CAD build for the part. Positions are in the model's coordinates, mm. Face numbers are marked on the shaded views. A direction names the side the tool comes from. Give positions to 0.01 mm unless a question says otherwise; leave off trailing zeros. Write each loop counter-clockwise with the first axis right and the second up, starting at its lowest first coordinate (ties: lowest second). Pieces come first, ordered by that corner, then holes. Notation, with made-up numbers: (-20, 65.5) - (17, 65.5) arc R23 ccw to (17, 97.5) - close; hole circle Ø3 at (-12, 27). An arc over 180 degrees is marked (long way). Answer as a JSON object with one key per item and string values.
from build123d import *

# Parameters (mm, degrees)
F0_W      = 24
F0_H      = 24
F1_DEPTH  = 6.5
F4_R      = 4
F5_R      = 1.35
F6_DEPTH  = 6.501
F8_DEPTH  = 5.5
F9_DEPTH  = 6.501
F10_DEPTH = 3.5


with BuildPart() as f1:
    # F0 (on Top) → F1 (new body)
    with BuildSketch(Plane.XY):
        with Locations((12, 12)):
            Rectangle(F0_W, F0_H)
    extrude(amount=F1_DEPTH)

    # F4
    f4_edges = [f1.edges().sort_by_distance(p)[0] for p in [
        (0, 0, 3.25),
        (24, 0, 3.25),
        (24, 24, 3.25),
        (0, 24, 3.25),
    ]]
    fillet(f4_edges, radius=F4_R)

    # F5 (on face) → F6 (cut, through all)
    with BuildSketch(Plane.XY.offset(6.5)):
        with Locations((4, 4)):
            Circle(F5_R)
        with Locations((4, 20)):
            Circle(F5_R)
        with Locations((20, 4)):
            Circle(F5_R)
        with Locations((20, 20)):
            Circle(F5_R)
    extrude(amount=-F6_DEPTH, mode=Mode.SUBTRACT)

    # F7 (on face) → F8 (cut, through all)
    with BuildSketch(Plane.XY.offset(6.5)):
        Polygon((16.1, 3.9), (16.1, 12), (16.1, 20.1), (7.9, 20.1), (7.9, 12), (7.9, 3.9), align=None)
        with BuildLine():
            Line((10.1, 9), (10.1, 15))
            ThreePointArc((10.1, 15), (12, 16.9), (13.9, 15))
            Line((13.9, 15), (13.9, 9))
            ThreePointArc((13.9, 9), (12, 7.1), (10.1, 9))
        make_face(mode=Mode.SUBTRACT)
    extrude(amount=-F8_DEPTH, mode=Mode.SUBTRACT)

    # F7 (on face) → F9 (cut, through all)
    with BuildSketch(Plane.XY.offset(6.5)):
        with BuildLine():
            ThreePointArc((13.9, 15), (12, 16.9), (10.1, 15))
            Line((10.1, 15), (10.1, 9))
            ThreePointArc((10.1, 9), (12, 7.1), (13.9, 9))
            Line((13.9, 9), (13.9, 15))
        make_face()
    extrude(amount=-F9_DEPTH, mode=Mode.SUBTRACT)

    # F7 (on face) → F10 (cut, through all)
    with BuildSketch(Plane.XY.offset(6.5)):
        Polygon((7.9, 12), (7.9, 20.1), (3.9, 16.1), (3.9, 12), (3.9, 7.9), (7.9, 3.9), align=None)
        Polygon((16.1, 20.1), (16.1, 12), (16.1, 3.9), (20.1, 7.9), (20.1, 12), (20.1, 16.1), align=None)
    extrude(amount=-F10_DEPTH, mode=Mode.SUBTRACT)


solid = f1.part
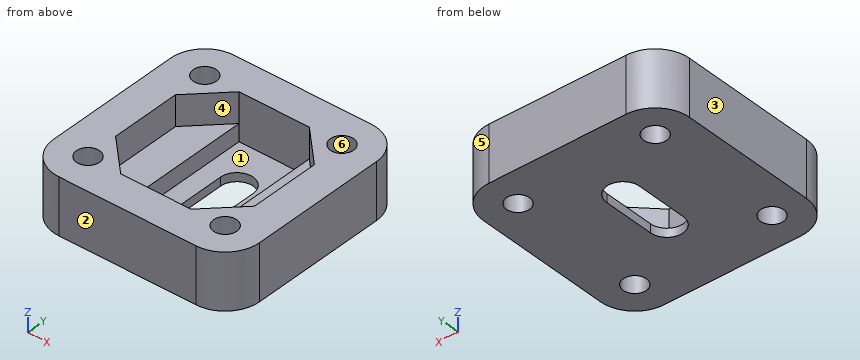
(1) Probe L1, parallel to Y at x = 4, z = 2.5; L2, parallel to Y at x = 20, z = 5; L3, parallel to X at y = 9.5, z = 0.5. List the from-to ranges inside material, lowest first. Write a range as [from, to].
Answer key:
{"L1": "y = [0, 2.65], [5.35, 18.65], [21.35, 24]", "L2": "y = [0, 2.65], [5.35, 7.8], [16.2, 18.65], [21.35, 24]", "L3": "x = [0, 10.1], [13.9, 24]"}
(2) Saw through at C-C, the plane y = 11.75. Give the cut face in (x, z).
Answer key:
{"outline": "(0, 0) - (10.1, 0) - (10.1, 1) - (7.9, 1) - (7.9, 3) - (3.9, 3) - (3.9, 6.5) - (0, 6.5) - close; (13.9, 0) - (24, 0) - (24, 6.5) - (20.1, 6.5) - (20.1, 3) - (16.1, 3) - (16.1, 1) - (13.9, 1) - close"}
(3) Saw through at B-B, the plane z = 4. Give the cut face in (x, y).
Answer key:
{"outline": "(0, 4) arc R4 ccw to (4, 0) - (20, 0) arc R4 ccw to (24, 4) - (24, 20) arc R4 ccw to (20, 24) - (4, 24) arc R4 ccw to (0, 20) - close; hole circle Ø2.7 at (4, 4); hole circle Ø2.7 at (4, 20); hole (3.9, 7.9) - (7.9, 3.9) - (16.1, 3.9) - (20.1, 7.9) - (20.1, 16.1) - (16.1, 20.1) - (7.9, 20.1) - (3.9, 16.1) - close; hole circle Ø2.7 at (20, 4); hole circle Ø2.7 at (20, 20)"}
(4) Pull direction Y, two halves, no side cores. Call the marked faces 3, 4, 5 and 6: pulls with the +Y half, pulls with the -Y half, needs draft (parallel to the pull), parting line crosses it, or undercut.
Answer key:
{"face 3": "needs draft", "face 4": "undercut", "face 5": "pulls with the +Y half", "face 6": "undercut"}
(5) Flat gauge pin, fed straight in: P1, Ø3, axis at x = 18, y = 11, coming from the +Z side. Where does the tip first touch, or does it go through?
Answer key:
{"P1": "stops at z = 3"}
(6) Saw through at A-A, the plane x = 12. Give the cut face in (y, z).
Answer key:
{"outline": "(0, 0) - (7.1, 0) - (7.1, 1) - (3.9, 1) - (3.9, 6.5) - (0, 6.5) - close; (16.9, 0) - (24, 0) - (24, 6.5) - (20.1, 6.5) - (20.1, 1) - (16.9, 1) - close"}
(7) Saw through at D-D, the plane y = 4.5. Give the cut face in (x, z), and give its area (3 significant figures).
Answer key:
{"outline": "(0, 0) - (2.75, 0) - (2.75, 6.5) - (0, 6.5) - close; (5.25, 0) - (18.75, 0) - (18.75, 6.5) - (16.7, 6.5) - (16.7, 3) - (16.1, 3) - (16.1, 1) - (7.9, 1) - (7.9, 3) - (7.3, 3) - (7.3, 6.5) - (5.25, 6.5) - close; (21.25, 0) - (24, 0) - (24, 6.5) - (21.25, 6.5) - close", "area": "74.1 mm²"}
(8) 3-axis set-ups, long thin cutter, end or side, ignore diameter. For the marked faces 1 and 2: which of +Z, -Z, +X, -X, +Y, -Y reach the whole face in a straight line?
Answer key:
{"face 1": "+Z", "face 2": "+Z, -Z, +X, -X, -Y"}
